Build history of the part. All positions in model axes, mm. A direction names the side the tool comes from. Round coordinates to 2 decimals unless told otherwise and drop trailing zeros. Order: outer loops, then holes, each group sorted by start corner. A loop starts at its lowest first (then second) coordinate and runs counter-clockwise, first axis right, second up. Notation, with made-up numbers: (30, 57) -> (83, 57) arc R26 cw to (83, 75) -> close; hole circle Ø8 at (80.5, 84). An arc over 180 degrees is marked (long way). Use a Markdown table: item, result. Add a question column.
Item 1: Slice it at C-C, the plane x = 1.75. Give the cut face in (y, z).
Item 2: Two-plate mould, pull along Y, no slides. Class faces 1 (the face through (0, -18, 0)), 2 (the face through (-10, -9, -7)), 3 (the face through (3, -17, 0)): released by +Y, released by -Y, zero draft, split by the parting line, or undercut.
Item 3: Pin check, flat tips, straight feed: pin 1 (4.5 mm diameter, centred on x = 5, z = 0, fed in from +Y); pin 2 (12 mm diameter, centred on y = -1, z = -7.5, fed in from -X); pin 3 (10 mm diameter, centred on x = 5, y = -8, fed in from +Z); pin 4 (3 mm diameter, centred on x = -5, z = 0, fed in from +Y). Stop position of each tip, or through.
Item 4: Probe L1, parallel to Y at x = 3, z = -12; L2, parallel to Z at x = 0, y = 7.5; L3, parallel to X at y = -16, z = 1.5. List the from-to ranges inside material, lowest first.
Item 5: 3-axis set-ups, long thin cutter, end or side, ignore diameter. For faces 4 (the face through (0, -15, 0)), 5 (the face through (-5, 15, -10)), 6 (the face through (-3.4, 10, -12.3)), 7 (the face through (0, -11, -11.3)): which of +Z, -Z, +X, -X, +Y, -Y reach the whole face in a straight line?
Item 6: Slice it at A-A, the plane z = 0. Give the cut face in (x, y).
Item 7: Slice it at D-D, the plane x = -5. Give the cut face in (y, z).
Item 8: Slice it at B-B, the plane y = -9. Give the cut face in (x, z), plus the area to 3 significant figures.
Autodesk Inventor part; units mm, degrees
ref_plane "YZ Plane" through (0, 0, 0) normal (1, 0, 0) x (0, 1, 0)
ref_plane "XZ Plane" through (0, 0, 0) normal (0, 1, 0) x (-1, 0, 0)
ref_plane "XY Plane" through (0, 0, 0) normal (0, 0, 1) x (1, 0, 0)
sketch "Sketch1" plane through (0, 0, 0) normal (0, 1, 0) x (-1, 0, 0)
  circle A0 centre (0, 0) radius 12.5
  circle A1 centre (0, 0) radius 11
  dimension "d0" = 25
  dimension "d1" = 22
extrude "Extrusion1" add sketch "Sketch1" along normal mid plane 30
sketch "Sketch2" plane through (0, 15, 0) normal (0, 1, 0) x (1, 0, 0)
  circle A0 centre (0, 0) radius 15
  circle A1 centre (0, 0) radius 12.5
  dimension "d4" = 30
extrude "Extrusion2" add sketch "Sketch2" against normal blind 5
sketch "Sketch3" plane through (0, -15, 0) normal (0, -1, 0) x (1, 0, 0)
  circle A0 centre (0, 0) radius 12.5
extrude "Extrusion3" add sketch "Sketch3" along normal blind 3
sketch "Sketch4" plane through (0, -18, 0) normal (0, -1, 0) x (1, 0, 0)
  line L0 (0, 0) -> (-5, 0)
  line L1 (0, 0) -> (5, 0)
  circle A0 centre (-5, 0) radius 2
  circle A1 centre (5, 0) radius 2
  dimension "d21" = 5
  dimension "d22" = 5
  dimension "d23" = 4
  dimension "d24" = 4
extrude "Extrusion4" cut sketch "Sketch4" against normal through all
sketch "Sketch6" plane through (0, 0, 0) normal (0, 0, 1) x (1, 0, 0)
  line L0 (-12.5, 10) -> (12.5, 10) construction
  line L1 (0, 10) -> (0, 0) construction
  line L2 (0, 0) -> (0, -9) construction
  line L3 (-12.5, -18) -> (12.5, -18) construction
  line L4 (0, -9) -> (-8, -9) construction
  line L5 (-8, -9) -> (8, -9) construction
  line L6 (-8, -11) -> (8, -11)
  line L7 (8, -7) -> (-8, -7)
  arc A0 (-8, -7) -> (-8, -11) centre (-8, -9) ccw
  arc A1 (8, -11) -> (8, -7) centre (8, -9) ccw
  dimension "d14" = 10
  dimension "d15" = 9
  dimension "d16" = 8
  dimension "d17" = 16
  dimension "d18" = 4
extrude "Extrusion6" cut sketch "Sketch6" against normal through all both and the other way through all
equation "\"d21\" = d22"
properties part number "EndEffectorRotational" material "ABS Plastic"
Check sheet entries:
| question | item | result |
|---|---|---|
| 1 | outline | (-18, -12.38) -> (-11, -12.38) -> (-11, -10.86) -> (-15, -10.86) -> (-15, 10.86) -> (-11, 10.86) -> (-11, 12.38) -> (-18, 12.38) -> close; (-7, -12.38) -> (10, -12.38) -> (10, -14.9) -> (15, -14.9) -> (15, -10.86) -> (-7, -10.86) -> close; (-7, 10.86) -> (15, 10.86) -> (15, 14.9) -> (10, 14.9) -> (10, 12.38) -> (-7, 12.38) -> close |
| 2 | face 1 | released by -Y |
| 2 | face 2 | undercut |
| 2 | face 3 | zero draft |
| 3 | pin 1 | y = -15 |
| 3 | pin 2 | x = -12.41 |
| 3 | pin 3 | z = 12.5 |
| 3 | pin 4 | through |
| 4 | L1 | -18 to -11, -7 to 15 |
| 4 | L2 | -12.5 to -11, 11 to 12.5 |
| 4 | L3 | -12.41 to -6.32, -3.68 to 3.68, 6.32 to 12.41 |
| 5 | face 4 | +Y |
| 5 | face 5 | +Z, -Z, +X, -X, +Y |
| 5 | face 6 | -Y |
| 5 | face 7 | +Z, -Z |
| 6 | outline | (-15, 10) -> (-12.5, 10) -> (-12.5, -18) -> (-7, -18) -> (-7, -15) -> (-11, -15) -> (-11, 15) -> (-15, 15) -> close; (-3, -18) -> (3, -18) -> (3, -15) -> (-3, -15) -> close; (7, -18) -> (12.5, -18) -> (12.5, 10) -> (15, 10) -> (15, 15) -> (11, 15) -> (11, -15) -> (7, -15) -> close |
| 7 | outline | (-18, -11.46) -> (-11, -11.46) -> (-11, -9.8) -> (-15, -9.8) -> (-15, -2) -> (-18, -2) -> close; (-18, 2) -> (-15, 2) -> (-15, 9.8) -> (-11, 9.8) -> (-11, 11.46) -> (-18, 11.46) -> close; (-7, -11.46) -> (10, -11.46) -> (10, -14.14) -> (15, -14.14) -> (15, -9.8) -> (-7, -9.8) -> close; (-7, 9.8) -> (15, 9.8) -> (15, 14.14) -> (10, 14.14) -> (10, 11.46) -> (-7, 11.46) -> close |
| 8 | outline | (-10, -7.5) -> (-10, -4.58) arc R11 cw to (-10, 4.58) -> (-10, 7.5) arc R12.5 ccw to start; (10, -7.5) arc R12.5 ccw to (10, 7.5) -> (10, 4.58) arc R11 cw to (10, -4.58) -> close |
| 8 | area | 38.8 mm2 |
